Build history of the part. All positions in model axes, mm. Round coordinates to 2 decimals unless told otherwise and drop trailing zeros. Order: outer loops, then holes, each group sorted by start corner. A loop starts at its lowest first (then second) coordinate and runs counter-clockwise, first axis right, second up. Notation, with made-up numbers: (-13.5, -1.75) -> (32.5, -1.75) arc R18 cw to (32.5, 17.25) -> close; hole circle Ø7 at (71, 23). An arc over 180 degrees is marked (long way). Use a Markdown table: item, result. Add a question column.
Item 1: Probe L1, parallel to X at y = 6, z = -406.4; L2, parallel to X at y = 2, z = -167; L3, parallel to Z at x = 195, y = 1.5. List the from-to ranges inside material, lowest first.
Item 2: Pin check, flat tips, straight feed: pin 1 (5 mm diameter, centred on y = 6, z = -55, fed in from -X); pin 2 (2 mm diameter, centred on x = 118.5, y = 11, fed in from -Z); pin 3 (14 mm diameter, centred on x = 0, z = -406.4, fed in from +Y); pin 4 (3 mm diameter, centred on x = 124, y = 9, fed in from -Z). Stop position of each tip, or through.
Item 3: Slice it at B-B, the plane x = 0. Give the cut face in (y, z) (3 decimals).
Item 4: Slice it at A-A, the plane y = 7.5. Give the cut face in (x, z), plus the area to 3 significant figures.
from build123d import *

# Parameters (mm, degrees)
SKETCH1_R           = 11.7094
BOSS_EXTRUDE1_DEPTH = 12.7
FILLET2_R           = 3.175
FILLET3_R           = 3.175


with BuildPart() as part:
    # Sketch1 → Boss-Extrude1 (new body)
    with BuildSketch(Plane(origin=(0, 0, 0), x_dir=(1, 0, 0), z_dir=(0, 1, 0))):
        with BuildLine():
            Line((134.815384615, 367.323076923), (271.584615385, 39.076923077))
            ThreePointArc((271.584615385, 39.076923077), (262.336309905, -56.357539936), (177.8, -101.6))
            Line((177.8, -101.6), (-177.8, -101.6))
            ThreePointArc((-177.8, -101.6), (-262.336309905, -56.357539936), (-271.584615385, 39.076923077))
            Line((-271.584615385, 39.076923077), (-134.815384615, 367.323076923))
            ThreePointArc((-134.815384615, 367.323076923), (0, 457.2), (134.815384615, 367.323076923))
        make_face()
        with Locations(Location((0, 406.4, 0), (0, 0, 270))):
            Circle(SKETCH1_R, mode=Mode.SUBTRACT)
    extrude(amount=BOSS_EXTRUDE1_DEPTH)

    # Fillet2
    fillet2_edges = [part.edges().sort_by_distance(p)[0] for p in [
        (-262.336309905, 12.7, 56.357539936),
        (0, 12.7, 101.6),
        (262.336309905, 12.7, 56.357539936),
        (203.2, 12.7, -203.2),
        (0, 12.7, -457.2),
        (-203.2, 12.7, -203.2),
    ]]
    fillet(fillet2_edges, radius=FILLET2_R)

    # Fillet3
    fillet3_edges = [part.edges().sort_by_distance(p)[0] for p in [
        (203.2, 0, -203.2),
        (262.336309905, 0, 56.357539936),
        (0, 0, 101.6),
        (-262.336309905, 0, 56.357539936),
        (-203.2, 0, -203.2),
        (0, 0, -457.2),
    ]]
    fillet(fillet3_edges, radius=FILLET3_R)


solid = part.part
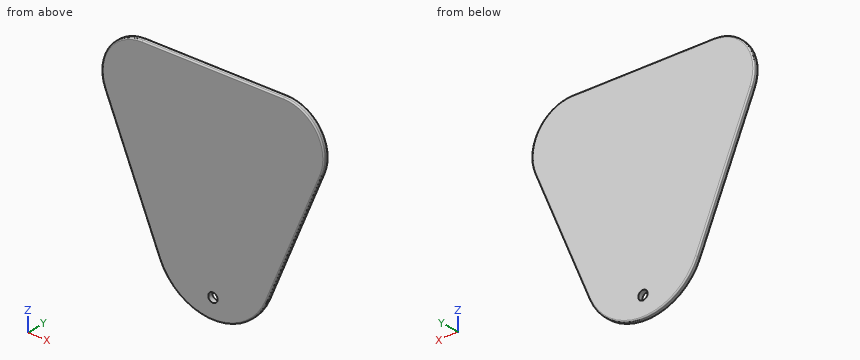
Check sheet entries:
| question | item | result |
|---|---|---|
| 1 | L1 | -110.72 to -11.71, 11.71 to 110.72 |
| 1 | L2 | -218.04 to 218.04 |
| 1 | L3 | -221.64 to 99.65 |
| 2 | pin 1 | x = -265.99 |
| 2 | pin 2 | z = -397.46 |
| 2 | pin 3 | through |
| 2 | pin 4 | z = -390.68 |
| 3 | outline | (0, -454.025) arc R3.175 ccw to (3.175, -457.2) -> (9.525, -457.2) arc R3.175 ccw to (12.7, -454.025) -> (12.7, -418.109) -> (0, -418.109) -> close; (0, -394.691) -> (12.7, -394.691) -> (12.7, 98.425) arc R3.175 ccw to (9.525, 101.6) -> (3.175, 101.6) arc R3.175 ccw to (0, 98.425) -> close |
| 4 | outline | (-271.58, -39.08) -> (-134.82, -367.32) arc R146.05 ccw to (134.82, -367.32) -> (271.58, -39.08) arc R101.6 ccw to (177.8, 101.6) -> (-177.8, 101.6) arc R101.6 ccw to start; hole circle Ø23.42 at (0, -406.4) |
| 4 | area | 224,000 mm2 |
